Can you work these out from the drawing? Everything is in mm from the part's minimum corner. A direction names the side the tool comes from. Round coordinates to 2 decimals unless told otherwise and drop trailing zeros. Order: outer loops, then holes, each group sorted by start corner. A loop starts at its lowest first (then second) coordinate and runs counter-clockwise, first axis right, second up. Notation, with made-up numbers: (27, 80.5) - (75, 80.5) arc R23 ccw to (75, 105.5) - close; hole circle Ø2 at (-24.5, 41.25). An arc over 180 degrees is marked (long way). Answer as a JSON object with one key per item and string values.
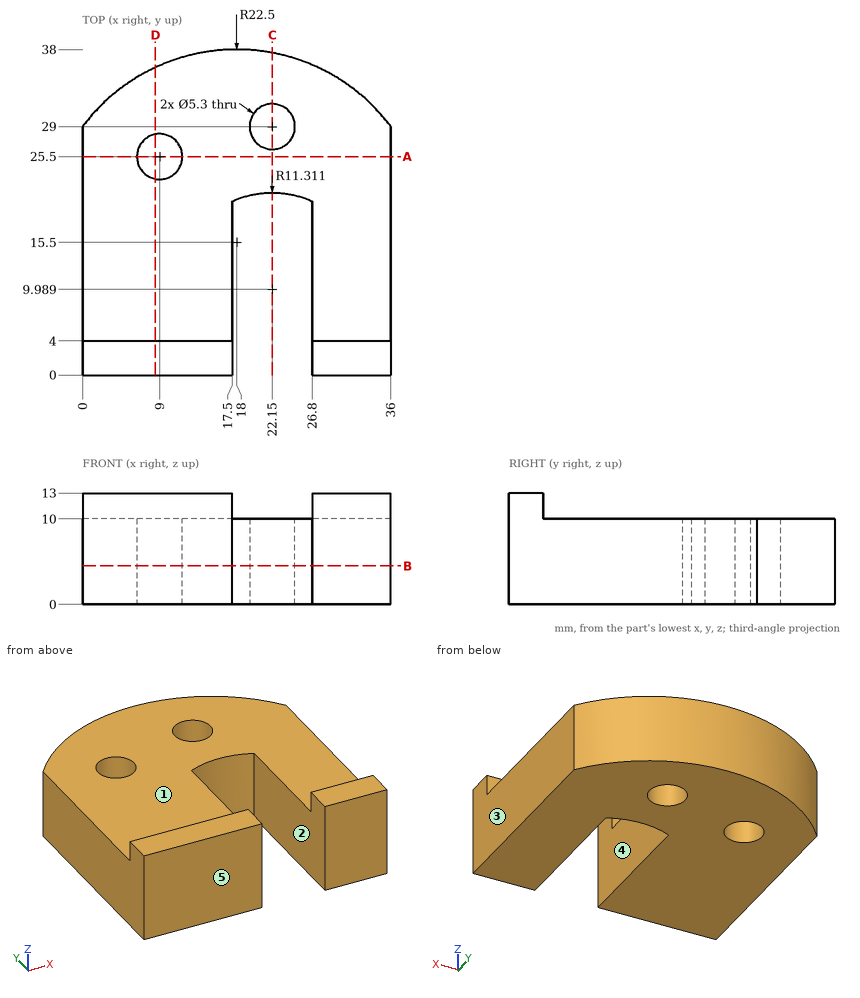
1. Imagine slicing it at B-B (z = 4.5). List the corners of the cut face in (x, y) for me.
Responses:
{"outline": "(0, 0) - (17.5, 0) - (17.5, 20.3) arc R11.31 cw to (26.8, 20.3) - (26.8, 0) - (36, 0) - (36, 29) arc R22.5 ccw to (0, 29) - close; hole circle Ø5.3 at (9, 25.5); hole circle Ø5.3 at (22.15, 29)"}
2. Imagine slicing it at A-A (y = 25.5). List the corners of the cut face in (x, z) for me, plus the area to 3 significant figures.
Responses:
{"outline": "(0, 0) - (6.35, 0) - (6.35, 10) - (0, 10) - close; (11.65, 0) - (36, 0) - (36, 10) - (11.65, 10) - close", "area": "307 mm2"}
3. For P1, Ø3.5, axis at x = 29.5, z = 12, coming from the +Y side; P2, Ø12, axis at x = 17, y = 23.5, coming from the +Z side; P3, Ø1, axis at y = 19, z = 11, coming from the -X side; P4, Ø2, axis at x = 26.5, z = 9.5, coming from the +Y side, each with a flat end and sliding along its axis, tell me the tip position at first contact or that it passes through.
Responses:
{"P1": "y = 4", "P2": "z = 10", "P3": "through", "P4": "y = 36.71"}
4. If I drill on L1, parallel to X at y = 17.5, z = 4.5; L2, parallel to Z at x = 8, y = 18; L3, parallel to Y at x = 22.15, z = 6, over which ranges is the centre line in solid material (lowest first)? Write a range as [from, to].
Responses:
{"L1": "[0, 17.5], [26.8, 36]", "L2": "[0, 10]", "L3": "[21.3, 26.35], [31.65, 37.61]"}
5. For the marked faces 4 and 5, which set-ups out of +Z, -Z, +X, -X, +Y, -Y let a thin tool reach every point of the face, with its end or its side?
Responses:
{"face 4": "+Z, -Z, -Y", "face 5": "+Z, -Z, +X, -X, -Y"}
6. Imagine slicing it at C-C (x = 22.15). List the corners of the cut face in (y, z) for me, plus the area to 3 significant figures.
Responses:
{"outline": "(21.3, 0) - (26.35, 0) - (26.35, 10) - (21.3, 10) - close; (31.65, 0) - (37.61, 0) - (37.61, 10) - (31.65, 10) - close", "area": "110 mm2"}
7. Imagine slicing it at D-D (x = 8.5). List the corners of the cut face in (y, z) for me, plus the area to 3 significant figures.
Responses:
{"outline": "(0, 0) - (22.9, 0) - (22.9, 10) - (4, 10) - (4, 13) - (0, 13) - close; (28.1, 0) - (35.9, 0) - (35.9, 10) - (28.1, 10) - close", "area": "319 mm2"}
8. Thinking about a two-plate mould opening in X: for the marked faces 1, 2 and 3, which applies, pulls with the +X half, pulls with the -X half, needs draft (parallel to the pull), parting line crosses it, or undercut?
Responses:
{"face 1": "needs draft", "face 2": "undercut", "face 3": "pulls with the +X half"}
